```python
from build123d import *

# Parameters (mm, degrees)
BOSS_EXTRUDE1_DEPTH = 5.08
SKETCH2_R           = 1.5875
CUT_EXTRUDE1_DEPTH  = 50.083323044
SKETCH3_R           = 1.5875
CUT_EXTRUDE2_DEPTH  = 50.083323044
CAVITY2_START       = -4.051115689
CAVITY2_OUTLINE_R   = 1.5875
CAVITY2_DEPTH       = 5.08
CUT_EXTRUDE3_DEPTH  = 50.083323044
SKETCH7_W           = 5.08
SKETCH7_H           = 11.047605328
CUT_EXTRUDE4_DEPTH  = 50.083323044


# Read off the part's stored shape, not the designer's step: Cavity2
with BuildPart() as part:
    # Sketch1 → Boss-Extrude1 (new body)
    with BuildSketch(Plane.XY):
        Polygon((-27.051, 40.64), (-16.891, 40.64), (-16.891, 35.56), (16.891, 35.56), (16.891, 40.64), (27.051, 40.64), (27.051, 30.48), (27.051, -40.64), (-27.051, -40.64), (-27.051, 30.48), align=None)
    extrude(amount=BOSS_EXTRUDE1_DEPTH)

    # Sketch2 → Cut-Extrude1 (cut, through all)
    with BuildSketch(Plane.XY.offset(5.08)):
        with Locations((-21.971, 38.1)):
            Circle(SKETCH2_R)
    extrude(amount=-CUT_EXTRUDE1_DEPTH, mode=Mode.SUBTRACT)

    # Sketch3 → Cut-Extrude2 (cut, through all)
    with BuildSketch(Plane(origin=(0, 0, 0), x_dir=(-1, 0, 0), z_dir=(0, 0, -1))):
        with Locations((-21.851181845, 37.741299139)):
            Circle(SKETCH3_R)
    extrude(amount=-CUT_EXTRUDE2_DEPTH, mode=Mode.SUBTRACT)

    # Cavity2 outline → Cavity2 (cut)
    with BuildSketch(Plane.YZ.offset(CAVITY2_START)):
        with BuildLine():
            ThreePointArc((-24.98622483, 5.08), (-25.105854872, 2.538856915), (-25.266867575, 0))
            Line((-25.266867575, 0), (-12.505553834, 0))
            ThreePointArc((-12.505553834, 0), (-11.65861771, 2.5332542), (-10.853159162, 5.08))
            Line((-10.853159162, 5.08), (-24.98622483, 5.08))
        make_face()
        with Locations((-18.473159162, 2.54)):
            Circle(CAVITY2_OUTLINE_R, mode=Mode.SUBTRACT)
    extrude(amount=CAVITY2_DEPTH, mode=Mode.SUBTRACT)

    # Sketch4 → Cut-Extrude3 (cut, through all)
    with BuildSketch(Plane.XY.offset(5.08)):
        Polygon((-4.051115689, -24.98622483), (-4.051115689, -23.553159162), (-6.591115689, -23.553159162), (-6.591115689, -5.773159162), (-27.051, 25.4), (-27.051, -40.64), (27.051, -40.64), (27.051, 25.4), (3.568884311, -5.773159162), (3.568884311, -23.553159162), (1.028884311, -23.553159162), (1.028884311, -24.98622483), align=None)
    extrude(amount=-CUT_EXTRUDE3_DEPTH, mode=Mode.SUBTRACT)

    # Sketch7 → Cut-Extrude4 (cut, through all)
    with BuildSketch(Plane(origin=(0, 0, 0), x_dir=(-1, 0, 0), z_dir=(0, 0, -1))):
        with Locations((1.511115689, -18.029356498)):
            Rectangle(SKETCH7_W, SKETCH7_H)
    extrude(amount=-CUT_EXTRUDE4_DEPTH, mode=Mode.SUBTRACT)


solid = part.part
```
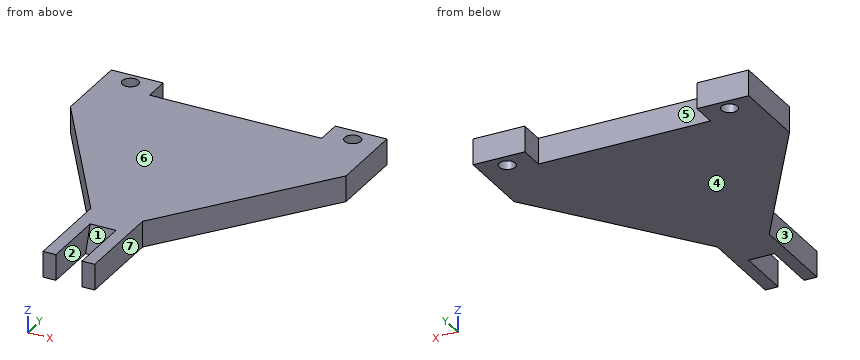
Read the model definition and answer for the solid it produces. Units are mm, in the model's axes. Face numbers are marked on the shaded views. A direction names the side the tool comes from. Give positions to 0.01 mm unless a question says otherwise; leave off trailing zeros. Order: outer loops, then holes, each group sorted by start corner. A loop starts at its lowest first (then second) coordinate and runs counter-clockwise, first axis right, second up.
(1) Find section A-A (y = -13.5). Give the vertices of the cut face in (x, z).
(2) Given pin 1 (1.5 mm diameter, centred on x = -3, z = 3.5, fed in from +Y); pin 2 (2.5 mm diameter, centred on y = -16.5, z = 2.5, fed in from -X); pin 3 (3 mm diameter, centred on y = -3.5, z = 0.5, fed in from -X); pin 4 (2 mm diameter, centred on x = -13.5, y = 33.5, fed in from -Z), each flat-ended and moving along its own axis, determine where each tip first touches the part or whether it passes through.
(3) Find section B-B (z = 1.9). Give the vertices of the cut face in (x, y) (1 decimal), plus the area to 3 significant figures.
(4) Find section D-D (x = 6). Give the vertices of the cut face in (y, z), plus the area to 3 significant figures.
(5) For a pull along X with two mould halves and no side action, classify the marked faces 1, 2, 3 and 4 as released by +X, released by -X, zero draft, split by the parting line, or undercut.
(6) Find section C-C (x = -3). Give the vertices of the cut face in (y, z).
(7) For the marked faces 5, 6 and 7, determine the directions among +Z, -Z, +X, -X, +Y, -Y from which every point of the face is accessible in a straight line to the end or side of a thin tool.
(8) Straight lines are drawn through the part: L1, parallel to X at y = -18, z = 2.3; L2, parallel to X at y = -10.5, z = 2; L3, parallel to Y at x = -5.5, z = 3.85. For each, find the intervals that lie inside material, in ascending order.
Result sheet:
1. outline: (-6.59, 0) - (-4.05, 0) - (-4.05, 5.08) - (-6.59, 5.08) - close; (1.03, 0) - (3.57, 0) - (3.57, 5.08) - (1.03, 5.08) - close
2. pin 1: stops at y = 35.56
2. pin 2: stops at x = -6.59
2. pin 3: stops at x = -9.07
2. pin 4: stops at z = 0
3. outline: (-27.1, 25.4) - (-6.6, -5.8) - (-6.6, -23.6) - (-4.1, -23.6) - (-4.1, -11.9) - (1, -11.9) - (1, -23.6) - (3.6, -23.6) - (3.6, -5.8) - (27.1, 25.4) - (27.1, 40.6) - (16.9, 40.6) - (16.9, 35.6) - (-16.9, 35.6) - (-16.9, 40.6) - (-27.1, 40.6) - close; hole circle Ø3.2 at (-22, 38.1); hole circle Ø3.2 at (21.9, 37.7)
3. area: 1,760 mm2
4. outline: (-2.55, 0) - (35.56, 0) - (35.56, 5.08) - (-2.55, 5.08) - close
4. area: 194 mm2
5. face 1: undercut
5. face 2: undercut
5. face 3: released by -X
5. face 4: zero draft
6. outline: (-12.51, 0) - (35.56, 0) - (35.56, 5.08) - (-10.85, 5.08) arc R163.58 cw to start
7. face 5: +Z, -Z, +Y
7. face 6: +Z, +X, -X, +Y, -Y
7. face 7: +Z, -Z, +X, -Y
8. L1: x = -6.59 to -4.05, 1.03 to 3.57
8. L2: x = -6.59 to 3.57
8. L3: y = -23.55 to 35.56
